Autodesk Inventor part; units mm, degrees
ref_plane "YZ Plane" through (0, 0, 0) normal (1, 0, 0) x (0, 1, 0)
ref_plane "XZ Plane" through (0, 0, 0) normal (0, 1, 0) x (-1, 0, 0)
ref_plane "XY Plane" through (0, 0, 0) normal (0, 0, 1) x (1, 0, 0)
sketch "Sketch1" plane through (0, 0, 0) normal (0, 0, 1) x (1, 0, 0)
  circle A0 centre (-2.6438, 6.9447) radius 6.8758
  line L0 (-9.4616, 7.8359) -> (-6.8245, 12.4034)
  line L1 (-6.8245, 1.4859) -> (-9.4616, 6.0534)
  line L2 (-0.0068, 0.5947) -> (-5.2808, 0.5947)
  line L3 (4.174, 6.0534) -> (1.537, 1.4859)
  line L4 (1.537, 12.4034) -> (4.174, 7.8359)
  line L5 (-5.2808, 13.2947) -> (-0.0068, 13.2947)
  point P0 (0, 0)
  point P1 (1.537, 1.4859)
  dimension "d0" = 13.7516
  dimension "d4" = 360
extrude "Extrusion1" add sketch "Sketch1" along normal blind 88.9 contours A0 L3 L2 L1 L0 L5 L4
sketch "Sketch2" plane through (0, 0, 88.9) normal (0, 0, 1) x (1, 0, 0)
  circle A0 centre (-2.6438, 6.9447) radius 2.5527
  line L0 (-5.2808, 0.5947) -> (-0.0068, 0.5947)
  line L1 (-2.6438, 6.9447) -> (-5.2808, 0.5947) construction
  line L2 (-2.6438, 6.9447) -> (-0.0068, 0.5947) construction
  point P0 (0, 0)
  dimension "d8" = 5.1054
  dimension "d9" = 6.35
extrude "Extrusion2" cut sketch "Sketch2" against normal blind 88.9
equation "\"d6\" = d5"
equation "\"d10\" = d5"
equation "\"d5\" = 88.9"
properties part number "AIntakeArmShaft" material "Aluminum 6061"
Part model, mm, in its own coordinate system. Round coordinates to 2 decimals unless told otherwise and drop trailing zeros. Loops run counter-clockwise (first coordinate to the right, second up) from the corner with the lowest first, then second, coordinate; pieces in that order, holes last.
1. Slice it at D-D (y = 2.75). Give the cut face in (x, z).
Solutions:
outline: (-7.55, 0) - (2.27, 0) - (2.27, 88.9) - (-7.55, 88.9) - close
2. Two-plate mould, pull along Y, no slides. Class faces 1 (the face through (2.874, 3.802, 43.828)), 2 (the face through (2.84, 10.15, 43.83)), 3 (the face through (-1.271, 9.097, 45.072)): pulls with the +Y half, pulls with the -Y half, needs draft (parallel to the pull), parting line crosses it, or undercut.
Solutions:
face 1: pulls with the -Y half
face 2: pulls with the +Y half
face 3: undercut
3. Drill centre lines: line 1 along X through (y, z) = (7.25, 75); line 2 along Y through (x, z) = (-2.5, 66.5); line 3 along X through (y, z) = (8.5, 64.5). Where is each one in solid material? Low to high.
Solutions:
line 1: x = -9.51 to -5.18, -0.11 to 4.23
line 2: y = 0.59 to 4.4, 9.49 to 13.29
line 3: x = -9.08 to -4.67, -0.62 to 3.79
4. Slice it at A-A (x = -1.5). Give the cut face in (y, z).
Solutions:
outline: (0.59, 0) - (4.66, 0) - (4.66, 88.9) - (0.59, 88.9) - close; (9.23, 0) - (13.29, 0) - (13.29, 88.9) - (9.23, 88.9) - close
5. Slice it at B-B (z = 31). Give the cut face in (x, y), and give its area (3 significant figures).
Solutions:
outline: (-9.46, 6.05) - (-6.82, 1.49) arc R6.88 ccw to (-5.28, 0.59) - (-0.01, 0.59) arc R6.88 ccw to (1.54, 1.49) - (4.17, 6.05) arc R6.88 ccw to (4.17, 7.84) - (1.54, 12.4) arc R6.88 ccw to (-0.01, 13.29) - (-5.28, 13.29) arc R6.88 ccw to (-6.82, 12.4) - (-9.46, 7.84) arc R6.88 ccw to start; hole circle Ø5.11 at (-2.64, 6.94)
area: 117 mm2
6. Slice it at C-C (x = -8.5). Give the cut face in (y, z).
Solutions:
outline: (4.39, 0) - (9.5, 0) - (9.5, 88.9) - (4.39, 88.9) - close
